For this review, take the finished solid that the model builds, in its own axes (mm). A direction names the side the tool comes from. Give positions to 0.01 mm unless a question says otherwise; leave off trailing zeros. Order: outer loops, then holes, each group sorted by start corner. A loop starts at its lowest first (then second) coordinate and runs counter-clockwise, first axis right, second up. Notation, with made-up numbers: M 9,44.25 L 47,44.25 A15 cw 47,70.25 Z; hole C 49.25,-16 d8. An arc over 180 degrees is marked long. Answer as CSV lines item,"result". Start each with the question number.
1. For line 1 along Y through (x, z) = (3, 22.5); line 2 along Z through (x, y) = (-38, -45.5); line 3 along X through (y, z) = (32, 50.5), list the stretches that pass through material, from the lowest coordinate up.
2. Mouldability with a two-part tool opening along X and no side actions: class faces 3 (the cylindrical face through (-56.1, -26.4, 49.3)), 4 (the flat face through (-51, 32, 100)), 5 (the flat face through (-43, -43, 10)) as pulls with the +X half, pulls with the -X half, needs draft (parallel to the pull), parting line crosses it, or undercut.
3. Clearance check with flat-ended pins moving along their axes: P1, Ø3, axis at x = 8, z = 34.5, coming from the +Y side; P2, Ø1.5, axis at x = 4, z = 35, coming from the +Y side; P3, Ø2, axis at x = -44, z = 21, coming from the -Y side. State where each tip first meets the part, or that it passes through.
4. We need section D-D, the plane y = 23.5. Give the boundary of the cut face in (x, z), and give its area (3 significant figures).
5. We need section B-B, the plane x = 14. Give the boundary of the cut face in (y, z), and give its area (3 significant figures).
6. Machinability: for faces 1 (the flat face through (23.179, 19.643, 0.986)), 2 (the flat face through (-43, -43, 90)), which of the approach directions +Z, -Z, +X, -X, +Y, -Y give a long, thin tool a straight path to every point of the face, cutting with its end or side? Answer none if there is none.
7. We need section A-A, the plane y = 0. Give the boundary of the cut face in (x, z).
from build123d import *

# Parameters (mm, degrees)
F0_W     = 5
F0_H     = 40
F0_W_2   = 40
F0_H_2   = 5
F1_DEPTH = 2
F2_DEPTH = 100
F5_DEPTH = 80


with BuildPart() as f1:
    # F0 (on Top) → F1 (new body)
    with BuildSketch(Plane.XY):
        with BuildLine():
            ThreePointArc((2.5, -59.9478940414), (43.3012701892, -41.5331193146), (60, 0))
            ThreePointArc((60, 0), (-41.5331193146, 43.3012701892), (-2.5, -59.9478940414))
            ThreePointArc((-2.5, -59.9478940414), (0, -60), (2.5, -59.9478940414))
        make_face()
        Polygon((-8.8388347648, -5.3033008589), (-5.3033008589, -8.8388347648), (-33.5875721064, -37.1231060123), (-37.1231060123, -33.5875721064), align=None, mode=Mode.SUBTRACT)
        with Locations((0, -30)):
            Rectangle(F0_W, F0_H, mode=Mode.SUBTRACT)
        Polygon((5.3033008589, -8.8388347648), (8.8388347648, -5.3033008589), (37.1231060123, -33.5875721064), (33.5875721064, -37.1231060123), align=None, mode=Mode.SUBTRACT)
        with Locations((-30, 0)):
            Rectangle(F0_W_2, F0_H_2, mode=Mode.SUBTRACT)
        Polygon((-5.3033008589, 8.8388347648), (-8.8388347648, 5.3033008589), (-37.1231060123, 33.5875721064), (-33.5875721064, 37.1231060123), align=None, mode=Mode.SUBTRACT)
        with Locations((30, 0)):
            Rectangle(F0_W_2, F0_H_2, mode=Mode.SUBTRACT)
        with Locations((0, 30)):
            Rectangle(F0_W, F0_H, mode=Mode.SUBTRACT)
        Polygon((8.8388347648, 5.3033008589), (5.3033008589, 8.8388347648), (33.5875721064, 37.1231060123), (37.1231060123, 33.5875721064), align=None, mode=Mode.SUBTRACT)
        with BuildLine():
            ThreePointArc((2.5, -59.9478940414), (0, -60), (-2.5, -59.9478940414))
            Line((-2.5, -59.9478940414), (-2.5, -61.9495762697))
            ThreePointArc((-2.5, -61.9495762697), (0, -62), (2.5, -61.9495762697))
            Line((2.5, -61.9495762697), (2.5, -59.9478940414))
        make_face()
        with BuildLine():
            ThreePointArc((-2.5, -59.9478940414), (-41.5331193146, 43.3012701892), (60, 0))
            ThreePointArc((60, 0), (43.3012701892, -41.5331193146), (2.5, -59.9478940414))
            Line((2.5, -59.9478940414), (2.5, -61.9495762697))
            ThreePointArc((2.5, -61.9495762697), (44.7157690306, -42.947642543), (62, 0))
            ThreePointArc((62, 0), (-42.947642543, 44.7157690306), (-2.5, -61.9495762697))
            Line((-2.5, -61.9495762697), (-2.5, -59.9478940414))
        make_face()
    extrude(amount=F1_DEPTH)

    # F0 (on Top) → F2 (join)
    with BuildSketch(Plane.XY):
        with BuildLine():
            ThreePointArc((2.5, -59.9478940414), (0, -60), (-2.5, -59.9478940414))
            Line((-2.5, -59.9478940414), (-2.5, -61.9495762697))
            ThreePointArc((-2.5, -61.9495762697), (0, -62), (2.5, -61.9495762697))
            Line((2.5, -61.9495762697), (2.5, -59.9478940414))
        make_face()
        with BuildLine():
            ThreePointArc((-2.5, -59.9478940414), (-41.5331193146, 43.3012701892), (60, 0))
            ThreePointArc((60, 0), (43.3012701892, -41.5331193146), (2.5, -59.9478940414))
            Line((2.5, -59.9478940414), (2.5, -61.9495762697))
            ThreePointArc((2.5, -61.9495762697), (44.7157690306, -42.947642543), (62, 0))
            ThreePointArc((62, 0), (-42.947642543, 44.7157690306), (-2.5, -61.9495762697))
            Line((-2.5, -61.9495762697), (-2.5, -59.9478940414))
        make_face()
    extrude(amount=F2_DEPTH)

    # F4 (on offset) → F5 (cut)
    with BuildSketch(Plane.XY.offset(10)):
        with BuildLine():
            ThreePointArc((2.5, -59.9478940414), (0, -59.80692448), (-2.5, -59.9478940414))
            Line((-2.5, -59.9478940414), (-2.5, -61.9495762697))
            ThreePointArc((-2.5, -61.9495762697), (0, -62.078494201), (2.5, -61.9495762697))
            Line((2.5, -61.9495762697), (2.5, -59.9478940414))
        make_face()
        with BuildLine():
            Line((-25.2507646861, -54.4279237411), (-26.0167753117, -56.2772369824))
            ThreePointArc((-26.0167753117, -56.2772369824), (-23.7564112369, -57.3530502014), (-21.3973776492, -58.1906541443))
            Line((-21.3973776492, -58.1906541443), (-20.6313670235, -56.3413409029))
            ThreePointArc((-20.6313670235, -56.3413409029), (-22.8871191392, -55.2543934295), (-25.2507646861, -54.4279237411))
        make_face()
        with BuildLine():
            Line((-44.1573293475, -40.6217954416), (-45.5727324249, -42.037198519))
            ThreePointArc((-45.5727324249, -42.037198519), (-43.8961242154, -43.8961242154), (-42.037198519, -45.5727324249))
            Line((-42.037198519, -45.5727324249), (-40.6217954416, -44.1573293475))
            ThreePointArc((-40.6217954416, -44.1573293475), (-42.2898818617, -42.2898818617), (-44.1573293475, -40.6217954416))
        make_face()
        with BuildLine():
            Line((-56.3413409029, -20.6313670235), (-58.1906541443, -21.3973776492))
            ThreePointArc((-58.1906541443, -21.3973776492), (-57.3530502014, -23.7564112369), (-56.2772369824, -26.0167753117))
            Line((-56.2772369824, -26.0167753117), (-54.4279237411, -25.2507646861))
            ThreePointArc((-54.4279237411, -25.2507646861), (-55.2543934295, -22.8871191392), (-56.3413409029, -20.6313670235))
        make_face()
        with BuildLine():
            Line((-59.9478940414, 2.5), (-61.9495762697, 2.5))
            ThreePointArc((-61.9495762697, 2.5), (-62.078494201, 0), (-61.9495762697, -2.5))
            Line((-61.9495762697, -2.5), (-59.9478940414, -2.5))
            ThreePointArc((-59.9478940414, -2.5), (-59.80692448, 0), (-59.9478940414, 2.5))
        make_face()
        with BuildLine():
            Line((20.6313670235, -56.3413409029), (21.3973776492, -58.1906541443))
            ThreePointArc((21.3973776492, -58.1906541443), (23.7564112369, -57.3530502014), (26.0167753117, -56.2772369824))
            Line((26.0167753117, -56.2772369824), (25.2507646861, -54.4279237411))
            ThreePointArc((25.2507646861, -54.4279237411), (22.8871191392, -55.2543934295), (20.6313670235, -56.3413409029))
        make_face()
        with BuildLine():
            Line((40.6217954416, -44.1573293475), (42.037198519, -45.5727324249))
            ThreePointArc((42.037198519, -45.5727324249), (43.8961242154, -43.8961242154), (45.5727324249, -42.037198519))
            Line((45.5727324249, -42.037198519), (44.1573293475, -40.6217954416))
            ThreePointArc((44.1573293475, -40.6217954416), (42.2898818617, -42.2898818617), (40.6217954416, -44.1573293475))
        make_face()
        with BuildLine():
            Line((54.4279237411, -25.2507646861), (56.2772369824, -26.0167753117))
            ThreePointArc((56.2772369824, -26.0167753117), (57.3530502014, -23.7564112369), (58.1906541443, -21.3973776492))
            Line((58.1906541443, -21.3973776492), (56.3413409029, -20.6313670235))
            ThreePointArc((56.3413409029, -20.6313670235), (55.2543934295, -22.8871191392), (54.4279237411, -25.2507646861))
        make_face()
        with BuildLine():
            Line((56.3413409029, 20.6313670235), (58.1906541443, 21.3973776492))
            ThreePointArc((58.1906541443, 21.3973776492), (57.3530502014, 23.7564112369), (56.2772369824, 26.0167753117))
            Line((56.2772369824, 26.0167753117), (54.4279237411, 25.2507646861))
            ThreePointArc((54.4279237411, 25.2507646861), (55.2543934295, 22.8871191392), (56.3413409029, 20.6313670235))
        make_face()
        with BuildLine():
            Line((44.1573293475, 40.6217954416), (45.5727324249, 42.037198519))
            ThreePointArc((45.5727324249, 42.037198519), (43.8961242154, 43.8961242154), (42.037198519, 45.5727324249))
            Line((42.037198519, 45.5727324249), (40.6217954416, 44.1573293475))
            ThreePointArc((40.6217954416, 44.1573293475), (42.2898818617, 42.2898818617), (44.1573293475, 40.6217954416))
        make_face()
        with BuildLine():
            Line((25.2507646861, 54.4279237411), (26.0167753117, 56.2772369824))
            ThreePointArc((26.0167753117, 56.2772369824), (23.7564112369, 57.3530502014), (21.3973776492, 58.1906541443))
            Line((21.3973776492, 58.1906541443), (20.6313670235, 56.3413409029))
            ThreePointArc((20.6313670235, 56.3413409029), (22.8871191392, 55.2543934295), (25.2507646861, 54.4279237411))
        make_face()
        with BuildLine():
            Line((2.5, 59.9478940414), (2.5, 61.9495762697))
            ThreePointArc((2.5, 61.9495762697), (0, 62.078494201), (-2.5, 61.9495762697))
            Line((-2.5, 61.9495762697), (-2.5, 59.9478940414))
            ThreePointArc((-2.5, 59.9478940414), (0, 59.80692448), (2.5, 59.9478940414))
        make_face()
        with BuildLine():
            Line((-20.6313670235, 56.3413409029), (-21.3973776492, 58.1906541443))
            ThreePointArc((-21.3973776492, 58.1906541443), (-23.7564112369, 57.3530502014), (-26.0167753117, 56.2772369824))
            Line((-26.0167753117, 56.2772369824), (-25.2507646861, 54.4279237411))
            ThreePointArc((-25.2507646861, 54.4279237411), (-22.8871191392, 55.2543934295), (-20.6313670235, 56.3413409029))
        make_face()
        with BuildLine():
            Line((-54.4279237411, 25.2507646861), (-56.2772369824, 26.0167753117))
            ThreePointArc((-56.2772369824, 26.0167753117), (-57.3530502014, 23.7564112369), (-58.1906541443, 21.3973776492))
            Line((-58.1906541443, 21.3973776492), (-56.3413409029, 20.6313670235))
            ThreePointArc((-56.3413409029, 20.6313670235), (-55.2543934295, 22.8871191392), (-54.4279237411, 25.2507646861))
        make_face()
        with BuildLine():
            Line((-40.6217954416, 44.1573293475), (-42.037198519, 45.5727324249))
            ThreePointArc((-42.037198519, 45.5727324249), (-43.8961242154, 43.8961242154), (-45.5727324249, 42.037198519))
            Line((-45.5727324249, 42.037198519), (-44.1573293475, 40.6217954416))
            ThreePointArc((-44.1573293475, 40.6217954416), (-42.2898818617, 42.2898818617), (-40.6217954416, 44.1573293475))
        make_face()
        with BuildLine():
            Line((59.9478940414, -2.5), (61.9495762697, -2.5))
            ThreePointArc((61.9495762697, -2.5), (62.078494201, 0), (61.9495762697, 2.5))
            Line((61.9495762697, 2.5), (59.9478940414, 2.5))
            ThreePointArc((59.9478940414, 2.5), (59.80692448, 0), (59.9478940414, -2.5))
        make_face()
    extrude(amount=F5_DEPTH, mode=Mode.SUBTRACT)


solid = f1.part
Result set:
1,line 1,"-61.93 to -59.92, 59.92 to 61.93"
1,line 2,"0 to 2"
1,line 3,"-53.1 to -50.75, 50.75 to 53.1"
2,face 3,"parting line crosses it"
2,face 4,"needs draft"
2,face 5,"undercut"
3,P1,"y = 61.66"
3,P2,"y = 61.91"
3,P3,"y = -41.46"
4,outline,"M -57.37,0 L -27.04,0 L -27.04,2 L -55.21,2 L -55.21,10 L -57.37,10 Z; M -57.37,90 L -55.21,90 L -55.21,100 L -57.37,100 Z; M -19.96,0 L -2.5,0 L -2.5,2 L -19.96,2 Z; M 2.5,0 L 19.96,0 L 19.96,2 L 2.5,2 Z; M 27.04,0 L 57.37,0 L 57.37,10 L 55.21,10 L 55.21,2 L 27.04,2 Z; M 55.21,90 L 57.37,90 L 57.37,100 L 55.21,100 Z"
4,area,"269 mm2"
5,outline,"M -60.4,0 L -17.54,0 L -17.54,2 L -58.34,2 L -58.34,100 L -60.4,100 Z; M -10.46,0 L -2.5,0 L -2.5,2 L -10.46,2 Z; M 2.5,0 L 10.46,0 L 10.46,2 L 2.5,2 Z; M 17.54,0 L 60.4,0 L 60.4,100 L 58.34,100 L 58.34,2 L 17.54,2 Z"
5,area,"606 mm2"
6,face 1,"+Z, -Z"
6,face 2,"none"
7,outline,"M -62,0 L -50,0 L -50,2 L -60,2 L -60,10 L -62,10 Z; M -62,90 L -60,90 L -60,100 L -62,100 Z; M -10,0 L 10,0 L 10,2 L -10,2 Z; M 50,0 L 62,0 L 62,10 L 60,10 L 60,2 L 50,2 Z; M 60,90 L 62,90 L 62,100 L 60,100 Z"
